Could you check a few things on this model? Use its own coordinates, in mm. Coordinates: 2 decimals unless noted, no trailing zeros. Loops run counter-clockwise (first coordinate to the right, second up) from the corner with the lowest first, then second, coordinate; pieces in that order, holes last.
Autodesk Inventor part; units mm, degrees
ref_plane "YZ Plane" through (0, 0, 0) normal (1, 0, 0) x (0, 1, 0)
ref_plane "XZ Plane" through (0, 0, 0) normal (0, 1, 0) x (-1, 0, 0)
ref_plane "XY Plane" through (0, 0, 0) normal (0, 0, 1) x (1, 0, 0)
sketch "Sketch2" plane through (0, 0, 0) normal (1, 0, 0) x (0, 1, 0)
  line L0 (0, 0) -> (0, 152.4)
  line L1 (0, 0) -> (-330.2, 0)
  line L2 (0, 152.4) -> (-342.9, 152.4)
  line L3 (-342.9, 152.4) -> (-342.9, 139.7) construction
  arc A0 (-342.9, 152.4) -> (-355.3918, 137.4098) centre (-342.9, 139.7) ccw
  line L4 (-330.2, 0) -> (-355.3918, 137.4098)
  point P0 (355.6, 152.4)
  dimension "d0" = 152.4
  dimension "d14" = 342.9
  dimension "d15" = 330.2
  dimension "d16" = 12.7
  dimension "d17" = 139.7
extrude "Extrusion1" add sketch "Sketch2" along normal blind 1290.32
properties part number "A" material "Granite, Cut, Polished"
(1) We'd pull the mould along Y, two halves only. Please class faces 1 (the face through (636, -169, 152.4)), 2 (the face through (636.13, -342.62, 67.74)), 3 (the face through (636, 0, 75)): +Y half, -Y half, draft (parallel to the pull), parting line (faces both ways), or undercut.
Answers:
face 1: draft
face 2: -Y half
face 3: +Y half
(2) Imagine slicing it at A-A, the plane x = 611. Write out the boundary of the cut face in (y, z), and give its area (3 significant figures).
Answers:
outline: (-355.39, 137.41) - (-330.2, 0) - (0, 0) - (0, 152.4) - (-342.9, 152.4) arc R12.7 ccw to start
area: 52,400 mm2
(3) For pin 1 (1.5 mm diameter, centred on x = 298.5, z = 59.5, fed in from -Y); pin 2 (3 mm diameter, centred on x = 141.5, z = 64.5, fed in from -Y); pin 3 (1 mm diameter, centred on x = 418.5, y = -127.5, fed in from -Z); pin 4 (8 mm diameter, centred on x = 144.5, z = 122, fed in from -Y), each with a flat end and sliding along its axis, tell me the tip position at first contact or that it passes through.
Answers:
pin 1: stops at y = -341.25
pin 2: stops at y = -342.3
pin 3: stops at z = 0
pin 4: stops at y = -353.3
(4) I need wall thicknesses on probe 1 along Y at (x, z) = (521.5, 141.5); probe 2 along Y at (x, z) = (151.5, 69). Which ranges of each line are inside material? Lowest first, please.
Answers:
probe 1: y = -355.47 to 0
probe 2: y = -342.85 to 0
(5) Imagine slicing it at B-B, the plane z = 12. Write out the boundary of the cut face in (x, y), and give its area (3 significant figures).
Answers:
outline: (0, -332.4) - (1290.32, -332.4) - (1290.32, 0) - (0, 0) - close
area: 429,000 mm2
